Can you work these out from the model? Positions are in its coordinate system, mm. A direction names the side the tool comes from. Coordinates: 2 decimals unless noted, no trailing zeros. Order: outer loops, then holes, each group sorted by start corner. A loop starts at its lowest first (then second) coordinate and runs counter-clockwise, first axis right, second up. Notation, with made-up numbers: (48, 30.25) -> (93, 30.25) arc R21 ccw to (93, 50.25) -> close; hole circle Ø8 at (2, 59.5). An arc over 180 degrees is marked (long way). Return JSON: item names as keys, results as strings. Group by question number.
1) If we section it at B-B, the plane x = 73: Please give me the cut outline in (y, z), then the cut area to 3 significant figures.
2) If we section it at C-C, the plane z = 79.5: Please give me the cut outline in (x, y) (3 decimals), then the cut area to 3 significant figures.
3) If I drill on probe 1 along Y at (x, z) = (75, 84); probe 2 along Z at (x, y) = (7.5, -6.5); probe 3 along Y at (x, z) = (116.8, -1), over which ranges is the centre line in solid material (lowest first)? Write a range as from..to.
4) For pin 1 (10.5 mm diameter, centred on x = 116.5, z = 4, fed in from -Y); pin 2 (3 mm diameter, centred on x = 60.5, y = -3, fed in from -Z); pin 3 (0.8 mm diameter, centred on x = 0.5, y = -24.5, fed in from +Z); pin 4 (1.1 mm diameter, centred on x = 6, z = -1, fed in from +Y), each with a flat end and sliding along its axis, tell me the tip position at first contact or that it passes through.
5) If we section it at A-A, the plane z = 94: Please give me the cut outline in (x, y), then the cut area to 3 significant figures.
6) Thinking about a two-plate mould opening in Z: for faces 6 (the flat face through (62.2, -0.3, 0)), 7 (the flat face through (0, -15, 46)), 8 (the cylindrical face through (8.713, -0.345, 112.164)), 9 (the flat face through (10.3, -13.3, -0.737)), which applies, +Z half, -Z half, draft (parallel to the pull), parting line (faces both ways), or undercut?
7) For faces 1 (the flat face through (62, -0.7, 59)), 2 (the flat face through (114.7, -13.1, -0.737)), 3 (the flat face through (0.7, -15, 46)), 4 (the flat face through (124.655, -13.243, 69.711)), 5 (the flat face through (124.7, -20.7, 4.5)), which set-ups out of +Z, -Z, +X, -X, +Y, -Y let a thin tool reach every point of the face, with its end or its side?
from build123d import *

# Parameters (mm, degrees)
SKETCH1_W                    = 125
SKETCH1_H                    = 120
BASE_FLANGE1_DEPTH           = 0.7
EDGE_FLANGE1_STRIP_W         = 4.2732
EDGE_FLANGE1_STRIP_H         = 0.7
EDGE_FLANGE1_STRIP_CUT_DEPTH = 120
EDGE_FLANGE1_DEPTH           = 120
EDGE_FLANGE1_FLAT_DEPTH      = 0.7
EDGE_FLANGE2_STRIP_W         = 4.2732
EDGE_FLANGE2_STRIP_H         = 0.7
EDGE_FLANGE2_STRIP_CUT_DEPTH = 120
EDGE_FLANGE2_DEPTH           = 120
EDGE_FLANGE2_FLAT_DEPTH      = 0.7
SKETCH10_R                   = 1.7
CUT_EXTRUDE1_DEPTH           = 10
EDGE_FLANGE3_DEPTH           = 15
EDGE_FLANGE4_DEPTH           = 15
F_6_CLEARANCE_HOLE1_D        = 3.7973
F_6_CLEARANCE_HOLE1_DEPTH    = 10
F_6_CLEARANCE_HOLE1_TIP      = 1.140824014
BREAK_CORNER1_START          = -1
BREAK_CORNER1_DEPTH          = 127
BREAK_CORNER1_START_2        = 123.5634
BREAK_CORNER1_2_DEPTH        = 2.4366
BREAK_CORNER1_START_3        = -2
BREAK_CORNER1_3_DEPTH        = 2
SKETCH23_W                   = 21.9
SKETCH23_H                   = 19.1
SKETCH23_W_2                 = 7.1
SKETCH23_H_2                 = 12.8
CUT_EXTRUDE2_DEPTH           = 0.7


with BuildPart() as part:
    # Base-Flange1: sheet metal written as solids
    # Sketch1 → Base-Flange1 (new body)
    with BuildSketch(Plane(origin=(0, 0, 0), x_dir=(1, 0, 0), z_dir=(0, 1, 0))):
        with Locations((62.5, -60)):
            Rectangle(SKETCH1_W, SKETCH1_H)
    extrude(amount=-BASE_FLANGE1_DEPTH)

    # Edge-Flange1: sheet metal written as solids
    # Edge-Flange1 strip (on a plane across the edge) → Edge-Flange1 strip cut (cut)
    with BuildSketch(Plane(origin=(125, -0.7, 0), x_dir=(-1, 0, 0), z_dir=(0, 0, 1))):
        with Locations((-0.7, -0.35)):
            Rectangle(EDGE_FLANGE1_STRIP_W, EDGE_FLANGE1_STRIP_H)
    extrude(amount=EDGE_FLANGE1_STRIP_CUT_DEPTH, mode=Mode.SUBTRACT)

    # Edge-Flange1 bend section (on a plane across the edge) → Edge-Flange1 (add)
    with BuildSketch(Plane(origin=(125, -0.7, 0), x_dir=(-1, 0, 0), z_dir=(0, 0, 1))):
        with BuildLine():
            Line((0, 0.7366), (0.7, 0.7366))
            ThreePointArc((0.7, 0.7366), (0.915745145, 0.215745145), (1.4366, 0))
            Line((1.4366, 0), (1.4366, -0.7))
            ThreePointArc((1.4366, -0.7), (0.420770398, -0.279229602), (0, 0.7366))
        make_face()
    extrude(amount=EDGE_FLANGE1_DEPTH)

    # Edge-Flange1 profile (on flange) → Edge-Flange1 flat (add)
    with BuildSketch(Plane(origin=(125, -0.7, 0), x_dir=(0, 0, 1), z_dir=(1, 0, 0))):
        Polygon((120, 0.7366), (120, 5), (20, 20), (0, 20), (0, 0.7366), align=None)
    extrude(amount=-EDGE_FLANGE1_FLAT_DEPTH)

    # Edge-Flange2: sheet metal written as solids
    # Edge-Flange2 strip (on a plane across the edge) → Edge-Flange2 strip cut (cut)
    with BuildSketch(Plane(origin=(0, -0.7, 120), x_dir=(1, 0, 0), z_dir=(0, 0, -1))):
        with Locations((-0.7, -0.35)):
            Rectangle(EDGE_FLANGE2_STRIP_W, EDGE_FLANGE2_STRIP_H)
    extrude(amount=EDGE_FLANGE2_STRIP_CUT_DEPTH, mode=Mode.SUBTRACT)

    # Edge-Flange2 bend section (on a plane across the edge) → Edge-Flange2 (add)
    with BuildSketch(Plane(origin=(0, -0.7, 120), x_dir=(1, 0, 0), z_dir=(0, 0, -1))):
        with BuildLine():
            Line((0, 0.7366), (0.7, 0.7366))
            ThreePointArc((0.7, 0.7366), (0.915745145, 0.215745145), (1.4366, 0))
            Line((1.4366, 0), (1.4366, -0.7))
            ThreePointArc((1.4366, -0.7), (0.420770398, -0.279229602), (0, 0.7366))
        make_face()
    extrude(amount=EDGE_FLANGE2_DEPTH)

    # Edge-Flange2 profile (on flange) → Edge-Flange2 flat (add)
    with BuildSketch(Plane(origin=(0, -0.7, 0), x_dir=(0, 0, 1), z_dir=(1, 0, 0))):
        Polygon((120, 0.7366), (120, 5), (55, 14.75), (55, 35), (0, 35), (0, 20), (0, 0.7366), align=None)
    extrude(amount=EDGE_FLANGE2_FLAT_DEPTH)

    # Sketch10 → Cut-Extrude1 (cut)
    with BuildSketch(Plane(origin=(0, 0, 0), x_dir=(1, 0, 0), z_dir=(0, 1, 0))):
        with Locations(Location((116.587265025, -113.862265027, 0), (0, 0, 270))):
            Circle(SKETCH10_R)
        with Locations(Location((116.587265025, -5.912265027, 0), (0, 0, 270))):
            Circle(SKETCH10_R)
        with Locations(Location((8.638202963, -6.362265027, 0), (0, 0, 270))):
            Circle(SKETCH10_R)
        with Locations(Location((8.638202963, -113.862265027, 0), (0, 0, 270))):
            Circle(SKETCH10_R)
    extrude(amount=-CUT_EXTRUDE1_DEPTH, mode=Mode.SUBTRACT)

    # Edge-Flange3: sheet metal written as solids
    # Edge-Flange3 section (on a plane across the edge) → Edge-Flange3 (add)
    with BuildSketch(Plane(origin=(124.3, -5.7, -0.7366), x_dir=(0, 0, 1), z_dir=(0, -1, 0))):
        with BuildLine():
            Line((-0.7, 0.7366), (-0.7, 15))
            Line((-0.7, 15), (0, 15))
            Line((0, 15), (0, 0.7366))
            ThreePointArc((0, 0.7366), (0.215745145, 0.215745145), (0.7366, 0))
            Line((0.7366, 0), (0.7366, -0.7))
            ThreePointArc((0.7366, -0.7), (-0.279229602, -0.279229602), (-0.7, 0.7366))
        make_face()
    extrude(amount=EDGE_FLANGE3_DEPTH)

    # Edge-Flange4: sheet metal written as solids
    # Edge-Flange4 section (on a plane across the edge) → Edge-Flange4 (add)
    with BuildSketch(Plane(origin=(0.7, -20.7, -0.7366), x_dir=(0, 0, 1), z_dir=(0, 1, 0))):
        with BuildLine():
            Line((-0.7, 0.7366), (-0.7, 15))
            Line((-0.7, 15), (0, 15))
            Line((0, 15), (0, 0.7366))
            ThreePointArc((0, 0.7366), (0.215745145, 0.215745145), (0.7366, 0))
            Line((0.7366, 0), (0.7366, -0.7))
            ThreePointArc((0.7366, -0.7), (-0.279229602, -0.279229602), (-0.7, 0.7366))
        make_face()
    extrude(amount=EDGE_FLANGE4_DEPTH)

    # #6 Clearance Hole1
    with Locations(Plane(origin=(0, 0, -1.4366), x_dir=(-1, 0, 0), z_dir=(0, 0, -1))):
        with Locations((-116.8, -13.2), (-8.2, -13.2)):
            Hole(F_6_CLEARANCE_HOLE1_D / 2, depth=F_6_CLEARANCE_HOLE1_DEPTH)
            with Locations((0, 0, -(F_6_CLEARANCE_HOLE1_DEPTH + F_6_CLEARANCE_HOLE1_TIP / 2))):  # 118° drill point
                Cone(0, F_6_CLEARANCE_HOLE1_D / 2, F_6_CLEARANCE_HOLE1_TIP, mode=Mode.SUBTRACT)

    # Break-Corner1: read off the stored shape, not the designer's step
    # Break-Corner1 outline → Break-Corner1 (cut)
    with BuildSketch(Plane.YZ.offset(BREAK_CORNER1_START)):
        with BuildLine():
            ThreePointArc((-6.01937233, 117.870851132), (-5.178422292, 119.394350526), (-3.547031448, 120))
            Line((-3.547031448, 120), (-5.7, 120))
            Line((-5.7, 120), (-6.01937233, 117.870851132))
        make_face()
        with BuildLine():
            ThreePointArc((-35.7, 52.5), (-34.967766953, 54.267766953), (-33.2, 55))
            Line((-33.2, 55), (-35.7, 55))
            Line((-35.7, 55), (-35.7, 52.5))
        make_face()
        with BuildLine():
            ThreePointArc((-33.2, 0), (-34.967766953, 0.732233047), (-35.7, 2.5))
            Line((-35.7, 2.5), (-35.7, 0))
            Line((-35.7, 0), (-33.2, 0))
        make_face()
    extrude(amount=BREAK_CORNER1_DEPTH, mode=Mode.SUBTRACT)

    # Break-Corner1 2 outline → Break-Corner1 2 (cut)
    with BuildSketch(Plane.YZ.offset(BREAK_CORNER1_START_2)):
        with BuildLine():
            ThreePointArc((-20.7, 19.813542987), (-20.693075631, 19.999483561), (-20.672340882, 20.184394119))
            Line((-20.672340882, 20.184394119), (-20.7, 20))
            Line((-20.7, 20), (-20.7, 19.813542987))
        make_face()
    extrude(amount=BREAK_CORNER1_2_DEPTH, mode=Mode.SUBTRACT)

    # Break-Corner1 3 outline → Break-Corner1 3 (cut)
    with BuildSketch(Plane.XY.offset(BREAK_CORNER1_START_3)):
        with BuildLine():
            ThreePointArc((13.2, -5.7), (14.967766953, -6.432233047), (15.7, -8.2))
            Line((15.7, -8.2), (15.7, -5.7))
            Line((15.7, -5.7), (13.2, -5.7))
        make_face()
        with BuildLine():
            ThreePointArc((15.7, -18.2), (14.967766953, -19.967766953), (13.2, -20.7))
            Line((13.2, -20.7), (15.7, -20.7))
            Line((15.7, -20.7), (15.7, -18.2))
        make_face()
        with BuildLine():
            ThreePointArc((111.8, -20.7), (110.032233047, -19.967766953), (109.3, -18.2))
            Line((109.3, -18.2), (109.3, -20.7))
            Line((109.3, -20.7), (111.8, -20.7))
        make_face()
        with BuildLine():
            ThreePointArc((109.3, -8.2), (110.032233047, -6.432233047), (111.8, -5.7))
            Line((111.8, -5.7), (109.3, -5.7))
            Line((109.3, -5.7), (109.3, -8.2))
        make_face()
    extrude(amount=BREAK_CORNER1_3_DEPTH, mode=Mode.SUBTRACT)

    # Sketch23 → Cut-Extrude2 (cut)
    with BuildSketch(Plane.ZY):
        with Locations((20, -18.5683)):
            Rectangle(SKETCH23_W, SKETCH23_H)
        with Locations((42, -18.5683)):
            Rectangle(SKETCH23_W_2, SKETCH23_H_2)
    extrude(amount=-CUT_EXTRUDE2_DEPTH, mode=Mode.SUBTRACT)


solid = part.part
Result sheet:
{
 "1": {"outline": "(-0.7, 0) -> (0, 0) -> (0, 120) -> (-0.7, 120) -> close", "area": "84.0 mm2"},
 "2": {"outline": "(0, -11.775) -> (0.7, -11.775) -> (0.7, -1.437) arc R0.737 cw to (1.437, -0.7) -> (123.563, -0.7) arc R0.737 cw to (124.3, -1.437) -> (124.3, -11.775) -> (125, -11.775) -> (125, -1.437) arc R1.437 ccw to (123.563, 0) -> (1.437, 0) arc R1.437 ccw to (0, -1.437) -> close", "area": "102 mm2"},
 "3": {"probe 1": "y = -0.7..0", "probe 2": "z = -1.44..-0.74", "probe 3": "y = -20.7..-15.1, -11.3..-5.7"},
 "4": {"pin 1": "stops at y = -20.7", "pin 2": "passes through", "pin 3": "stops at z = 55", "pin 4": "stops at y = -5.7"},
 "5": {"outline": "(0, -9.6) -> (0.7, -9.6) -> (0.7, -1.44) arc R0.74 cw to (1.44, -0.7) -> (123.56, -0.7) arc R0.74 cw to (124.3, -1.44) -> (124.3, -9.6) -> (125, -9.6) -> (125, -1.44) arc R1.44 ccw to (123.56, 0) -> (1.44, 0) arc R1.44 ccw to (0, -1.44) -> close", "area": "99.3 mm2"},
 "6": {"face 6": "-Z half", "face 7": "draft", "face 8": "undercut", "face 9": "+Z half"},
 "7": {"face 1": "+Z, -Z, -Y", "face 2": "+Z, +Y, -Y", "face 3": "+Z, -Y", "face 4": "+Z, +X, -Y", "face 5": "+Z, -Z, +X, -Y"}
}
